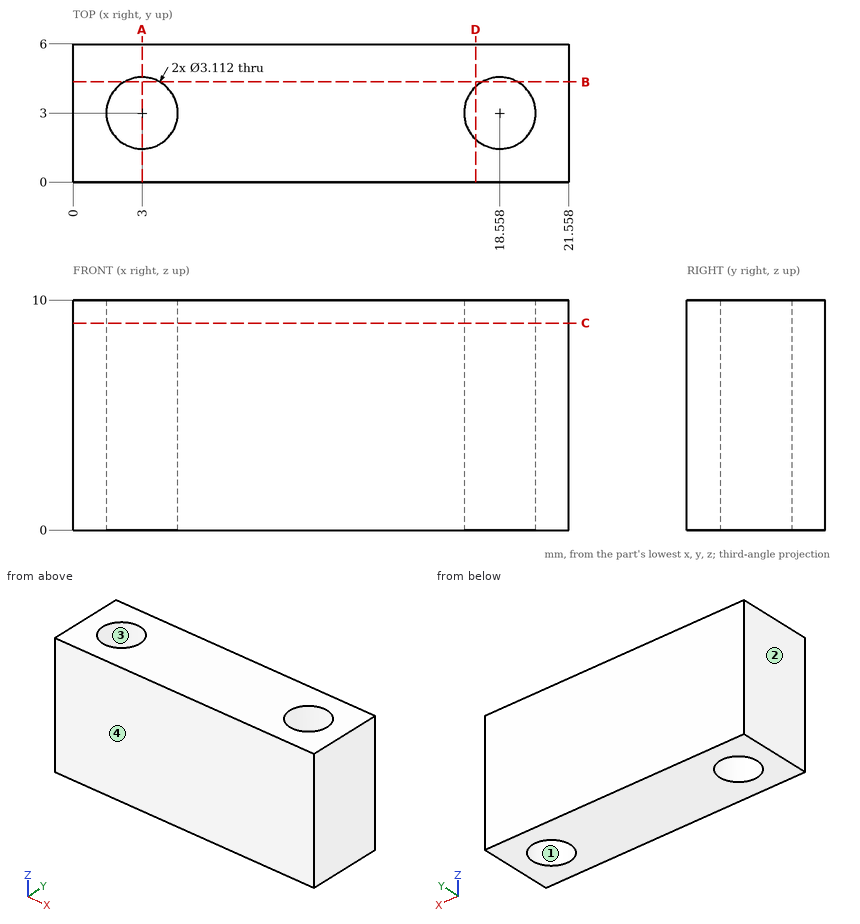
Geometry: see drawing. Coordinates: mm, zero at the bounding-box minimum. Coordinates: 2 decimals unless noted, no trailing zeros. Write each loop counter-clockwise with the first axis right and the second up, starting at its lowest first coordinate (ties: lowest second). Pieces come first, ordered by that corner, then holes. Notation, with made-up numbers: (65, 36.25) - (98, 36.25) arc R16 ccw to (98, 56.25) - close; hole circle Ø5 at (37, -33). An arc over 180 degrees is marked (long way). Put each result on its own line as item: value. Start each with the question number.
1) Mould query, pull axis Y, two halves, no side actions, for the marked faces 1, 2, 3 and 4. Classes: pulls with the +Y half, pulls with the -Y half, needs draft (parallel to the pull), parting line crosses it, or undercut.
2) Cut plane D-D (x = 17.5). Return the cut outline in (y, z).
3) Cut plane A-A (x = 3). Return the cut outline in (y, z) (1 decimal).
4) Cut plane C-C (z = 9). Return the cut outline in (x, y) (1 decimal).
5) Contact query for a flat-ended pin moving along its axis: pin 1 (3 mm diameter, centred on x = 3, y = 3, fed in from -Z). Output: stop coordinate, or through.
6) Ray query, L1, parallel to X at y = 2.05, z = 5.25 (1 decimal); L2, parallel to Y at x = 3, z = 4.5 (1 decimal); L3, parallel to X at y = 2.45, z = 2.5 (1 decimal). Return the intervals inside material, ascending.
7) Cut plane B-B (y = 4.35). Return the cut outline in (x, z) (1 decimal), plus the area to 3 significant figures.
Resolved:
1. face 1: undercut
1. face 2: needs draft
1. face 3: undercut
1. face 4: pulls with the -Y half
2. outline: (0, 0) - (1.86, 0) - (1.86, 10) - (0, 10) - close; (4.14, 0) - (6, 0) - (6, 10) - (4.14, 10) - close
3. outline: (0, 0) - (1.4, 0) - (1.4, 10) - (0, 10) - close; (4.6, 0) - (6, 0) - (6, 10) - (4.6, 10) - close
4. outline: (0, 0) - (21.6, 0) - (21.6, 6) - (0, 6) - close; hole circle Ø3.1 at (3, 3); hole circle Ø3.1 at (18.6, 3)
5. pin 1: passes through
6. L1: x = 0 to 1.8, 4.2 to 17.3, 19.8 to 21.6
6. L2: y = 0 to 1.4, 4.6 to 6
6. L3: x = 0 to 1.5, 4.5 to 17.1, 20 to 21.6
7. outline: (0, 0) - (2.2, 0) - (2.2, 10) - (0, 10) - close; (3.8, 0) - (17.8, 0) - (17.8, 10) - (3.8, 10) - close; (19.3, 0) - (21.6, 0) - (21.6, 10) - (19.3, 10) - close
7. area: 185 mm2
